The listing builds one solid part. Answer for the finished solid, in the listing's coordinates (mm). A direction names the side the tool comes from. Round coordinates to 2 decimals unless told otherwise and drop trailing zeros. Write each loop counter-clockwise with the first axis right and the second up, starting at its lowest first coordinate (ties: lowest second). Pieces come first, ordered by that corner, then holes.
Item 1: Each of these flat-tipped pins is pushed along its axis until it touches: pin 1 (17.5 mm diameter, centred on x = 0, y = 0, fed in from +Z); pin 2 (4 mm diameter, centred on x = 32.5, y = -24.6, fed in from +Z); pin 3 (5 mm diameter, centred on x = 39.5, z = 7, fed in from +Y); pin 4 (2 mm diameter, centred on y = 8.5, z = 2.5, fed in from -X). Where does it stop, or does it pass through?
Item 2: Find the intervals of material crossed by probe 1 along X at (y, z) = (-15.5, 7.1); probe 2 along Y at (x, z) = (-15.5, 7.55); probe 3 along X at (y, z) = (15.5, 6.2), in increasing order.
Item 3: Find section D-D on z = 8. Give the vertices of the cut face in (x, y).
Item 4: Find section A-A on y = 0. Give the vertices of the cut face in (x, z), then the cut area to 3 significant figures.
Item 5: For a pull along Y with two mould halves and no side action, classify faces 4 (the face through (-42.5, -24, 5)), 5 (the face through (0, 22.5, 5)), 6 (the face through (-17, 15.57, 6.96)) as +Y half, -Y half, draft (parallel to the pull), parting line (faces both ways), or undercut.
Item 6: Find section C-C on x = 0. Give the vertices of the cut face in (y, z).
Item 7: Find section B-B on y = 15.5. Give the vertices of the cut face in (x, z).
Item 8: A tool of negligible diameter and unlimited length cuts with its end or side. For faces 1 (the face through (38, -14.6, 5)), 2 (the face through (14, -17, 4)), 3 (the face through (2, -5, 6)), from which of +Z, -Z, +X, -X, +Y, -Y can it reach the whole face along a straight path? Write none if from no direction.
```python
from build123d import *

# Parameters (mm, degrees)
SKETCH1_R           = 1.5
SKETCH1_R_2         = 2.5
SKETCH1_R_3         = 5
BOSS_EXTRUDE1_DEPTH = 10
SKETCH2_R           = 11
CUT_EXTRUDE1_DEPTH  = 4
CHAMFER1_SIZE       = 10
SKETCH3_R           = 2.85
CUT_EXTRUDE2_DEPTH  = 4


with BuildPart() as part:
    # Sketch1 → Boss-Extrude1 (new body)
    with BuildSketch(Plane.XY):
        Polygon((22.5, 22.5), (-22.5, 22.5), (-22.5, -14.6), (-42.5, -14.6), (-42.5, -34.6), (42.5, -34.6), (42.5, -14.6), (22.5, -14.6), align=None)
        with Locations((-15.5, 15.5)):
            Circle(SKETCH1_R, mode=Mode.SUBTRACT)
        with Locations((15.5, 15.5)):
            Circle(SKETCH1_R, mode=Mode.SUBTRACT)
        with Locations((32.5, -24.6)):
            Circle(SKETCH1_R_2, mode=Mode.SUBTRACT)
        with Locations((-32.5, -24.6)):
            Circle(SKETCH1_R_2, mode=Mode.SUBTRACT)
        Circle(SKETCH1_R_3, mode=Mode.SUBTRACT)
        with Locations((15.5, -15.5)):
            Circle(SKETCH1_R, mode=Mode.SUBTRACT)
        with Locations((-15.5, -15.5)):
            Circle(SKETCH1_R, mode=Mode.SUBTRACT)
    extrude(amount=BOSS_EXTRUDE1_DEPTH)

    # Sketch2 → Cut-Extrude1 (cut)
    with BuildSketch(Plane.XY.offset(10)):
        Circle(SKETCH2_R)
    extrude(amount=-CUT_EXTRUDE1_DEPTH, mode=Mode.SUBTRACT)

    # Chamfer1
    chamfer1_edges = [part.edges().sort_by_distance(p)[0] for p in [
        (22.5, -14.6, 5),
        (-22.5, -14.6, 5),
    ]]
    chamfer(chamfer1_edges, length=CHAMFER1_SIZE)

    # Sketch3 → Cut-Extrude2 (cut)
    with BuildSketch(Plane(origin=(0, 0, 0), x_dir=(-1, 0, 0), z_dir=(0, 0, -1))):
        with Locations((-15.5, 15.5)):
            Circle(SKETCH3_R)
        with Locations((15.5, 15.5)):
            Circle(SKETCH3_R)
        with Locations((-15.5, -15.5)):
            Circle(SKETCH3_R)
        with Locations((15.5, -15.5)):
            Circle(SKETCH3_R)
    extrude(amount=-CUT_EXTRUDE2_DEPTH, mode=Mode.SUBTRACT)


solid = part.part
```
Check values:
1. pin 1: stops at z = 6
1. pin 2: passes through
1. pin 3: stops at y = -14.6
1. pin 4: stops at x = -22.5
2. probe 1: x = -42.5 to -17, -14 to 14, 17 to 42.5
2. probe 2: y = -34.6 to -17, -14 to 14, 17 to 22.5
2. probe 3: x = -22.5 to -17, -14 to 14, 17 to 22.5
3. outline: (-42.5, -34.6) - (42.5, -34.6) - (42.5, -14.6) - (32.5, -14.6) - (22.5, -4.6) - (22.5, 22.5) - (-22.5, 22.5) - (-22.5, -4.6) - (-32.5, -14.6) - (-42.5, -14.6) - close; hole circle Ø5 at (-32.5, -24.6); hole circle Ø3 at (-15.5, -15.5); hole circle Ø3 at (-15.5, 15.5); hole circle Ø22 at (0, 0); hole circle Ø3 at (15.5, -15.5); hole circle Ø3 at (15.5, 15.5); hole circle Ø5 at (32.5, -24.6)
4. outline: (-22.5, 0) - (-5, 0) - (-5, 6) - (-11, 6) - (-11, 10) - (-22.5, 10) - close; (5, 0) - (22.5, 0) - (22.5, 10) - (11, 10) - (11, 6) - (5, 6) - close
4. area: 302 mm2
5. face 4: draft
5. face 5: +Y half
5. face 6: undercut
6. outline: (-34.6, 0) - (-5, 0) - (-5, 6) - (-11, 6) - (-11, 10) - (-34.6, 10) - close; (5, 0) - (22.5, 0) - (22.5, 10) - (11, 10) - (11, 6) - (5, 6) - close
7. outline: (-22.5, 0) - (-18.35, 0) - (-18.35, 4) - (-17, 4) - (-17, 10) - (-22.5, 10) - close; (-14, 4) - (-12.65, 4) - (-12.65, 0) - (12.65, 0) - (12.65, 4) - (14, 4) - (14, 10) - (-14, 10) - close; (17, 4) - (18.35, 4) - (18.35, 0) - (22.5, 0) - (22.5, 10) - (17, 10) - close
8. face 1: +Z, -Z, +X, +Y
8. face 2: -Z
8. face 3: +Z
